Design review of the part built by this model. Coordinates are the model's own, in mm. Face numbers are marked on the shaded views. Round coordinates to 2 decimals unless told otherwise and drop trailing zeros. Order: outer loops, then holes, each group sorted by start corner. A loop starts at its lowest first (then second) coordinate and runs counter-clockwise, first axis right, second up.
from build123d import *

# Parameters (mm, degrees)
F1_DEPTH        = 20.5
F2_W            = 200
F2_H            = 20
F3_DEPTH        = 20.5
F4_DEPTH        = 19
F5_DEPTH        = 25
F6_DEPTH        = 25
F9_D            = 6.6
F9_CBORE_D      = 14
F9_CBORE_DEPTH  = 8
F11_D           = 6.8
F11_CBORE_D     = 14
F11_CBORE_DEPTH = 8
F12_DEPTH       = 0.5


with BuildPart() as f1:
    # F0 (on Front) → F1 (new body)
    with BuildSketch(Plane.XZ):
        Polygon((42.4411185086, 149.9418458194), (-157.5588814914, 149.9418458194), (-87.5588814914, -26.0581541806), (-57.5588814914, -26.0581541806), (-27.5588814914, -26.0581541806), align=None)
    extrude(amount=F1_DEPTH)

    # F2 (on face) → F3 (join)
    with BuildSketch(Plane.XZ.offset(20.5)):
        with Locations((-57.5588814914, 159.9418458194)):
            Rectangle(F2_W, F2_H)
    extrude(amount=-F3_DEPTH)

    # F4 (cut): a face of the model
    f4_faces = [f1.faces().sort_by_distance(p)[0] for p in [
        (-57.5588814914, -10.25, -26.0581541806),
    ]]
    extrude(f4_faces, amount=-F4_DEPTH, mode=Mode.SUBTRACT)

    # F5 (cut): a face of the model
    f5_faces = [f1.faces().sort_by_distance(p)[0] for p in [
        (-87.5588814914, -10.25, -16.5581541806),
    ]]
    extrude(f5_faces, amount=-F5_DEPTH, mode=Mode.SUBTRACT)

    # F6 (cut): a face of the model
    f6_faces = [f1.faces().sort_by_distance(p)[0] for p in [
        (-27.5588814914, -10.25, -16.5581541806),
    ]]
    extrude(f6_faces, amount=-F6_DEPTH, mode=Mode.SUBTRACT)

    # F9 (through all)
    with Locations(Plane.XZ.offset(20.5)):
        with Locations((-72.5584090471, 58.9418458194), (-42.5584090471, 58.9418458194), (-42.5584090471, 12.9418458194), (-72.5584090471, 12.9418458194)):
            CounterBoreHole(F9_D / 2, F9_CBORE_D / 2, F9_CBORE_DEPTH)

    # F11 (through all)
    with Locations(Plane.XZ.offset(20.5)):
        with Locations((-141.5588814914, 160.9418458194), (26.4411185086, 160.9418458194), (-57.5588814914, 160.9418458194)):
            CounterBoreHole(F11_D / 2, F11_CBORE_D / 2, F11_CBORE_DEPTH)

    # F12 (cut): a face of the model
    f12_faces = [f1.faces().sort_by_distance(p)[0] for p in [
        (-57.5588840418, 0, 95.3321481764),
    ]]
    extrude(f12_faces, amount=-F12_DEPTH, mode=Mode.SUBTRACT)


solid = f1.part
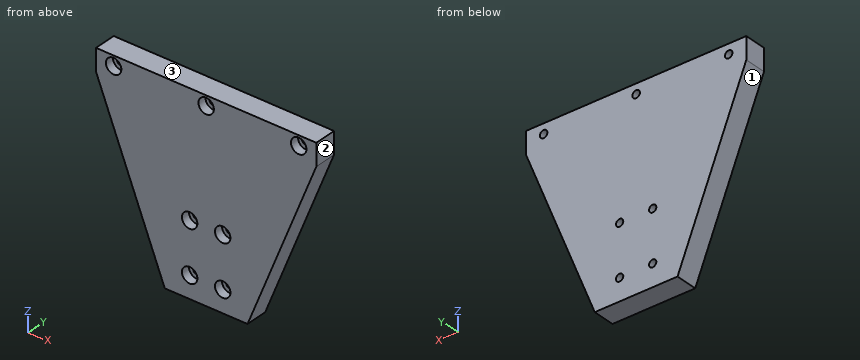
1) The part is to be moulded in two halves that separate along Z. For the marked faces 1, 2 and 3, say which applies: released by +Z, released by -Z, zero draft, split by the parting line, or undercut.
Results:
face 1: released by -Z
face 2: zero draft
face 3: released by +Z
2) Take a section at B-B on z = 111. Give the boundary of the cut face in (x, y).
Results:
outline: (-142.07, -20.5) - (26.95, -20.5) - (26.95, -0.5) - (-142.07, -0.5) - close
3) Clearance check with flat-ended pins moving along their axes: P1, Ø4, axis at x = -72.56, z = 12.94, coming from the +Y side; P2, Ø11, axis at x = -42.5, z = 11.5, coming from the -Y side; P3, Ø4, axis at y = -6.5, z = 42.5, coming from the +X side. State where each tip first meets the part, or that it passes through.
Results:
P1: passes through
P2: stops at y = -12.5
P3: stops at x = 0.5
4) Take a section at C-C on x = 16.5. Give the boundary of the cut face in (y, z).
Results:
outline: (-20.5, 84.72) - (-0.5, 84.72) - (-0.5, 169.94) - (-20.5, 169.94) - close
5) Take a section at A-A on y = -9.5. Give the boundary of the cut face in (x, z), plus the area to 3 significant figures.
Results:
outline: (-157.56, 149.94) - (-95.12, -7.06) - (-20, -7.06) - (42.44, 149.94) - (42.44, 169.94) - (-157.56, 169.94) - close; hole circle Ø6.8 at (-141.56, 160.94); hole circle Ø6.6 at (-72.56, 12.94); hole circle Ø6.6 at (-72.56, 58.94); hole circle Ø6.8 at (-57.56, 160.94); hole circle Ø6.6 at (-42.56, 12.94); hole circle Ø6.6 at (-42.56, 58.94); hole circle Ø6.8 at (26.44, 160.94)
area: 25,400 mm2
6) To check wall thickness, follow line 1 along X through (y, z) = (-6.75, 13.5); line 2 along X through (y, z) = (-9.5, 10); line 3 along Z through (x, y) = (-58, -15.25). State the ranges of each line that lie inside material, in increasing order.
Results:
line 1: x = -103.29 to -75.81, -69.31 to -45.81, -39.31 to -11.83
line 2: x = -101.9 to -74.05, -71.06 to -44.05, -41.06 to -13.22
line 3: z = -7.06 to 153.96, 167.93 to 169.94
